Verification items for this drawing (mm, ordinates from the low corner). A direction names the side the tool comes from. Coordinates: 2 decimals unless noted, no trailing zeros. Loops run counter-clockwise (first coordinate to the right, second up) from the corner with the lowest first, then second, coordinate; pieces in that order, holes last. Notation, with made-up numbers: M -3.5,59 L 46.5,59 A10 cw 46.5,68 Z; hole C 49.5,32 d6. An arc over 180 degrees is marked long. One line per question, with ' | ' between items. Start each with the question number.
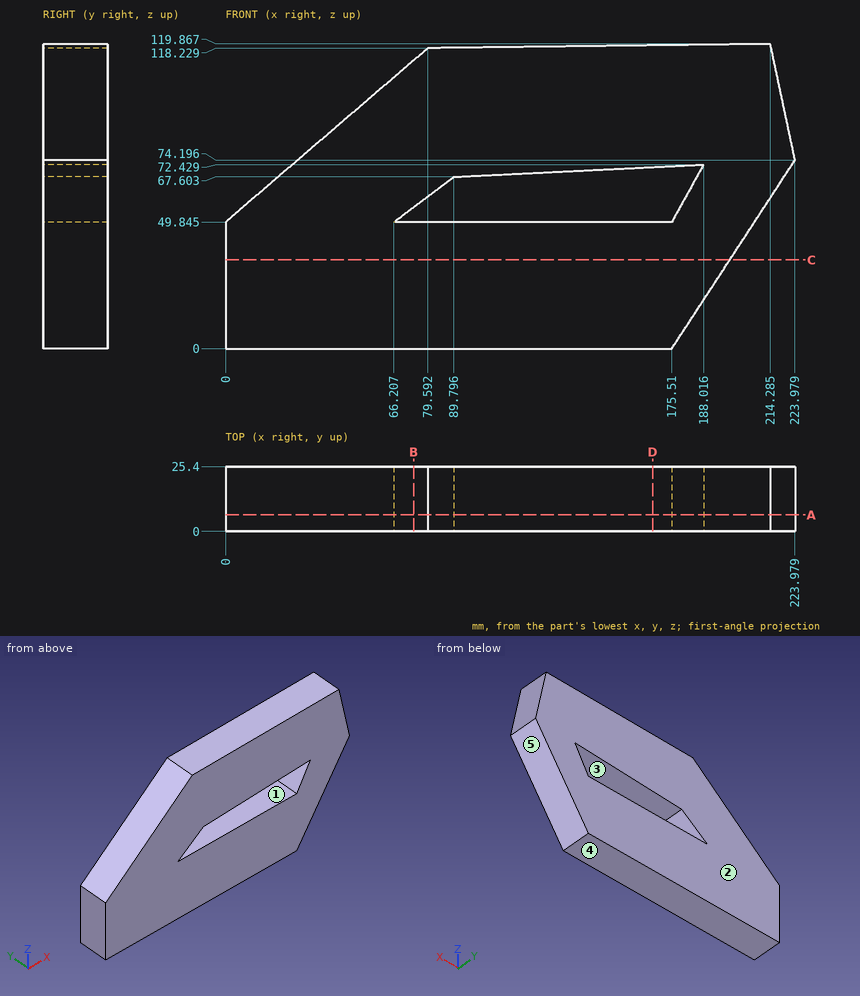
1. Draft check along X on the marked faces 3, 4 and 5. Enter one of: +X half, -X half, draft (parallel to the pull), parting line (faces both ways), or undercut.
2. Depth check by flat-ended pin: pin 1 Ø2 at (x, y) = (99, 3) entering from +Z; pin 2 Ø5 at (y, z) = (20, 73.5) entering from -X; pin 3 Ø5 at (y, z) = (12, 72) entering from +X; pin 4 Ø1.5 at (x, y) = (126, 2.5) entering from +Z. Enter the tip coordinate at first touch or a pass-through.
3. Thickness scan on line 1 (Z direction, x = 137, y = 21.75) (1 decimal); line 2 (Z direction, x = 161.5, y = 4.75) (1 decimal); line 3 (X direction, y = 7.5, z = 41) (1 decimal). Record the ranges inside material, lowest first.
4. Sectioned sample at D-D (x = 168). Record the cut outline in (y, z) (1 decimal).
5. Tool access check on the marked faces 1 and 2. Record the directions out of +Z, -Z, +X, -X, +Y, -Y that give a thin tool (end or side, any length) a straight path to the whole face; none if there is none.
6. Sectioned sample at B-B (x = 74). Record the cut outline in (y, z) (1 decimal), and give its area (3 significant figures).
7. Sectioned sample at A-A (y = 6.5). Record the cut outline in (x, z) (1 decimal).
8. Sectioned sample at C-C (z = 35). Record the cut outline in (x, y), and give its area (3 significant figures).
Result:
1) face 3: undercut | face 4: draft | face 5: +X half
2) pin 1: stops at z = 118.48 | pin 2: stops at x = 24.62 | pin 3: stops at x = 223.98 | pin 4: stops at z = 118.8
3) line 1: z = 0 to 49.8, 69.9 to 118.9 | line 2: z = 0 to 49.8, 71.1 to 119.2 | line 3: x = 0 to 202.3
4) outline: M 0,0 L 25.4,0 L 25.4,49.8 L 0,49.8 Z; M 0,71.4 L 25.4,71.4 L 25.4,119.3 L 0,119.3 Z
5) face 1: +Y, -Y | face 2: +Z, -Z, +X, -X, +Y
6) outline: M 0,0 L 25.4,0 L 25.4,49.8 L 0,49.8 Z; M 0,55.7 L 25.4,55.7 L 25.4,113.4 L 0,113.4 Z | area: 2,730 mm2
7) outline: M 0,0 L 175.5,0 L 224,74.2 L 214.3,119.9 L 79.6,118.2 L 0,49.8 Z; hole M 66.2,49.8 L 175.5,49.8 L 188,72.4 L 89.8,67.6 Z
8) outline: M 0,0 L 198.37,0 L 198.37,25.4 L 0,25.4 Z | area: 5,040 mm2
